Geometry check sheet. Reference: the model listing, model coordinates, mm. A direction names the side the tool comes from. Coordinates: 2 decimals unless noted, no trailing zeros. Write each loop counter-clockwise with the first axis right and the second up, starting at its lowest first coordinate (ties: lowest second). Pieces come first, ordered by that corner, then holes. Notation, with made-up numbers: M 37,36.25 L 85,36.25 A28 ccw 85,72.25 Z; hole C 33.25,80.25 d2. An arc over 180 degrees is marked long. Put each result on its own line as item: value. Start each with the question number.
1) Scan lines: line 1 along X through (y, z) = (28, -0.25); line 2 along X through (y, z) = (25.5, 0.25); line 3 along Y through (x, z) = (-10.25, -7.25). Record each from-to range of solid material in increasing order.
2) Cross-section at C-C on x = 5.75. Record the cut outline in (y, z), plus the area to 3 significant figures.
3) Cross-section at A-A on z = 0. Record the cut outline in (x, y).
4) Mould release check, pull along X, two halves, no side actions. Record for faces 5 (the flat face through (-7.073, 14.79, -5.659)), 6 (the flat face through (-5.659, 14.79, 7.073)), 7 (the flat face through (7, 30, 0)), 8 (the cylindrical face through (0.66, 28.479, -14.985)): released by +X, released by -X, zero draft, split by the parting line, or undercut.
5) Set-up check for faces 1 (the cylindrical face through (2.956, 10.14, -11.285)), 2 (the flat face through (-8, 0, 0)), 3 (the cylindrical face through (-11.05, 16.31, 5.74)), 4 (the flat face through (0, 15, 6.55)): record each of +Z, -Z, +X, -X, +Y, -Y from which the full face is reachable in a straight line by a thin tool's end or side.
6) Gauge pin test, flat ends, axial feed: pin 1 (1 mm diameter, centred on x = -9.5, y = 15.5, fed in from +Z); pin 2 (1.5 mm diameter, centred on y = 11.5, z = -10.5, fed in from -X); pin 3 (1.5 mm diameter, centred on y = 7.5, z = 3, fed in from +X). Record the tip position at first contact, or that the pin passes through.
7) Cross-section at B-B on y = 20.75. Record the cut outline in (x, z), plus the area to 3 significant figures.
from build123d import *

# Parameters (mm, degrees)
SKETCH1_R           = 12.45
BOSS_EXTRUDE3_DEPTH = 30
BOSS_EXTRUDE4_START = -3
SKETCH4_R           = 15
SKETCH4_R_2         = 12.45
BOSS_EXTRUDE4_DEPTH = 3
CUT_EXTRUDE1_DEPTH  = 20
FILLET1_R           = 4


with BuildPart() as part:
    # Sketch1 → Boss-Extrude3 (new body)
    with BuildSketch(Plane(origin=(0, 0, 0), x_dir=(1, 0, 0), z_dir=(0, 1, 0))):
        with Locations(Location((0, 0, 0), (0, 0, 270))):
            Circle(SKETCH1_R)
        Polygon((6.196446609, 7.610660172), (7.610660172, 6.196446609), (6.55, 5.135786438), (6.55, -5.135786438), (7.610660172, -6.196446609), (6.196446609, -7.610660172), (5.135786438, -6.55), (-5.135786438, -6.55), (-6.196446609, -7.610660172), (-7.610660172, -6.196446609), (-6.55, -5.135786438), (-6.55, 5.135786438), (-7.610660172, 6.196446609), (-6.196446609, 7.610660172), (-5.135786438, 6.55), (5.135786438, 6.55), align=None, mode=Mode.SUBTRACT)
    extrude(amount=BOSS_EXTRUDE3_DEPTH)

    # Sketch4 → Boss-Extrude4 (add)
    with BuildSketch(Plane(origin=(0, 30, 0), x_dir=(1, 0, 0), z_dir=(0, 1, 0)).offset(BOSS_EXTRUDE4_START)):
        with Locations(Location((0, 0, 0), (0, 0, 270))):
            Circle(SKETCH4_R)
        with Locations(Location((0, 0, 0), (0, 0, 270))):
            Circle(SKETCH4_R_2, mode=Mode.SUBTRACT)
    extrude(amount=BOSS_EXTRUDE4_DEPTH)

    # Sketch5 → Cut-Extrude1 (cut)
    with BuildSketch(Plane.XZ):
        with BuildLine():
            Line((4.135786438, -11.742988144), (4.135786438, 11.742988144))
            ThreePointArc((4.135786438, 11.742988144), (12.45, 0), (4.135786438, -11.742988144))
        make_face()
    extrude(amount=-CUT_EXTRUDE1_DEPTH, mode=Mode.SUBTRACT)

    # Fillet1
    fillet1_edges = [part.edges().sort_by_distance(p)[0] for p in [
        (4.135786438, 10, -11.742988144),
        (4.135786438, 10, 11.742988144),
    ]]
    fillet(fillet1_edges, radius=FILLET1_R)


solid = part.part
Answer key:
1. line 1: x = -15 to -6.55, 6.55 to 15
1. line 2: x = -12.45 to -6.55, 6.55 to 12.45
1. line 3: y = 27 to 30
2. outline: M 20,-11.04 L 27,-11.04 L 27,-13.85 L 30,-13.85 L 30,-7.16 L 20,-7.16 Z; M 20,7.16 L 30,7.16 L 30,13.85 L 27,13.85 L 27,11.04 L 20,11.04 Z
2. area: 94.4 mm²
3. outline: M -15,27 L -12.45,27 L -12.45,0 L -6.55,0 L -6.55,30 L -15,30 Z; M 6.55,20 L 12.45,20 L 12.45,27 L 15,27 L 15,30 L 6.55,30 Z
4. face 5: undercut
4. face 6: undercut
4. face 7: zero draft
4. face 8: split by the parting line
5. face 1: -Z, +X, -Y
5. face 2: +Z, -Z, +X, -X, -Y
5. face 3: -Y
5. face 4: +Y, -Y
6. pin 1: stops at z = 8.6
6. pin 2: stops at x = -7.74
6. pin 3: stops at x = -6.55
7. outline: C 0,0 d24.9; hole M -7.61,-6.2 L -6.2,-7.61 L -5.14,-6.55 L 5.14,-6.55 L 6.2,-7.61 L 7.61,-6.2 L 6.55,-5.14 L 6.55,5.14 L 7.61,6.2 L 6.2,7.61 L 5.14,6.55 L -5.14,6.55 L -6.2,7.61 L -7.61,6.2 L -6.55,5.14 L -6.55,-5.14 Z
7. area: 307 mm²
